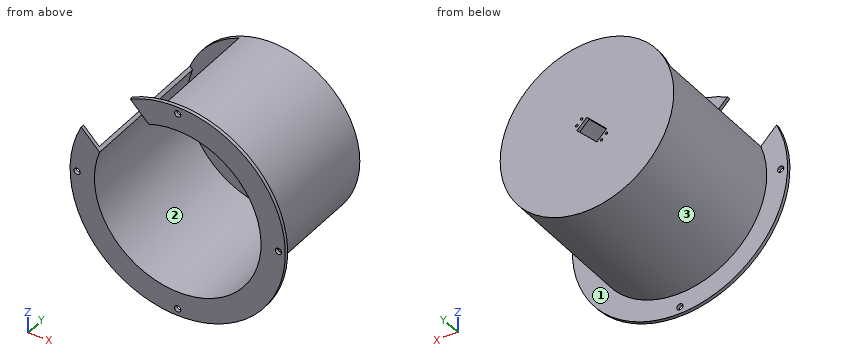
Autodesk Inventor part; units mm, degrees
ref_plane "Work Plane2" through (-109.6016, 0, 109.6016) normal (0.7071, 0, -0.7071) x (0, 1, 0)
ref_plane "XZ Plane" through (0, 0, 0) normal (0, 1, 0) x (-1, 0, 0)
ref_plane "XY Plane" through (0, 0, 0) normal (0, 0, 1) x (1, 0, 0)
sketch "Sketch1" plane through (0, 0, 0) normal (0, 1, 0) x (-1, 0, 0)
  circle A0 centre (0, 0) radius 120
  circle A1 centre (0, 0) radius 125
  circle A2 centre (0, 0) radius 155
  dimension "d0" = 240
  dimension "d1" = 250
  dimension "d2" = 310
extrude "Extrusion1" add sketch "Sketch1" along normal blind 205 contours A0 | A1 | A2
sketch "Sketch3" plane through (0, 205, 0) normal (0, 1, 0) x (1, 0, 0)
  circle A0 centre (0, 0) radius 155
  circle A1 centre (0, 0) radius 125
  dimension "d27" = 250
  dimension "d28" = 310
extrude "Extrusion3" cut sketch "Sketch3" against normal blind 200
sketch "Sketch4" plane through (0, 5, 0) normal (0, 1, 0) x (1, 0, 0)
  circle A0 centre (0, 145) radius 4.5
  circle A1 centre (0, 0) radius 155
  line L0 (0, 155) -> (0, 125)
  circle A2 centre (0, 0) radius 125
  circle A3 centre (-145, 0) radius 4.5
  line L1 (-155, 0) -> (-125, 0)
  circle A4 centre (0, -145) radius 4.5
  line L2 (0, -155) -> (0, -125)
  circle A5 centre (145, 0) radius 4.5
  line L3 (155, 0) -> (125, 0)
  dimension "d31" = 9
  dimension "d32" = 0
  dimension "d33" = 145
  dimension "d36" = 360
extrude "Extrusion4" cut sketch "Sketch4" against normal through all contours A0 L0 | L0 A0 | L3 A5 | A5 L3 | L1 A3 | A3 L1 | L2 A4 | A4 L2
sketch "Sketch5" plane through (0, 0, 0) normal (0, -1, 0) x (1, 0, 0)
  circle A0 centre (0, 0) radius 120
  dimension "d40" = 240
extrude "Extrusion5" cut sketch "Sketch5" against normal blind 200
ref_plane "Work Plane2" through (-109.6016, 0, 109.6016) normal (0.7071, 0, -0.7071) x (0, 1, 0)
ref_plane "Work Plane1" through (0, 0, 0) normal (0.7071, 0, -0.7071) x (0, 1, 0)
sketch "Sketch6" plane through (-109.6016, 0, 109.6016) normal (0.7071, 0, -0.7071) x (0, 1, 0)
  line L0 (0, -50) -> (200, -50)
  line L1 (200, -50) -> (200, 50)
  line L2 (200, 50) -> (0, 50)
  line L3 (0, 50) -> (0, -50)
  line L4 (0, 155) -> (0, -155)
  line L5 (-41, 0) -> (246, 0)
  point P0 (0, 0)
  dimension "d44" = 200
  dimension "d45" = 100
  dimension "d46" = 0
  dimension "d47" = 50
extrude "Extrusion6" cut sketch "Sketch6" along normal up to surface
sketch "Sketch7" plane through (0, 205, 0) normal (0, 1, 0) x (1, 0, 0)
  circle A0 centre (0, 0) radius 10
  line L0 (0, 0) -> (31, 0) construction
  line L1 (7.0711, 7.0711) -> (-14.2128, 28.355)
  line L2 (-14.2128, 28.355) -> (-28.355, 14.2128)
  line L3 (-28.355, 14.2128) -> (-7.0711, -7.0711)
  line L4 (-7.0711, -7.0711) -> (0.2828, -14.425)
  line L5 (-7.0711, -7.0711) -> (3.3289, -7.0711) construction
  line L6 (0.2828, -14.425) -> (14.425, -0.2828)
  line L7 (14.425, -0.2828) -> (7.0711, 7.0711)
  circle A1 centre (-28.0368, 20.9657) radius 1.75
  circle A2 centre (-20.9657, 28.0368) radius 1.75
  circle A3 centre (7.6721, -14.7432) radius 1.75
  circle A4 centre (14.7432, -7.6721) radius 1.75
  dimension "d50" = 20
  dimension "d53" = 20
  dimension "d55" = 10.4
  dimension "d56" = 45
  dimension "d57" = 30.1
  dimension "d58" = 3.5
  dimension "d61" = 5
  dimension "d65" = 10
  dimension "d68" = 50.5
  dimension "d71" = 4.55
extrude "Extrusion7" cut sketch "Sketch7" against normal through all
properties part number "mechanism_cover"
Geometry check sheet. Reference: the model listing, model coordinates, mm. Face numbers are marked on the shaded views. Give positions to 0.01 mm unless a question says otherwise; leave off trailing zeros. Loops run counter-clockwise (first coordinate to the right, second up) from the corner with the lowest first, then second, coordinate; pieces in that order, holes last. Notation, with made-up numbers: M 66,-25 L 90,-25 A12 cw 90,-18 Z; hole C 64,29 d9. An arc over 180 degrees is marked long. Answer as a JSON object with one key per item and string values. Group by question number.
Item 1: Sectioned sample at A-A on z = -145. Record the boundary of the cut face in (x, y), plus the area to 3 significant figures.
Item 2: Sectioned sample at B-B on x = 145. Record the boundary of the cut face in (y, z).
Item 3: Material ranges on L1, parallel to X at y = 2, z = 0; L2, parallel to Z at x = 0, y = 112.5, recorded low to high.
Item 4: Mould release check, pull along X, two halves, no side actions. Record for the marked faces 1, 2 and 3: pulls with the +X half, pulls with the -X half, needs draft (parallel to the pull), parting line crosses it, or undercut.
Item 5: Sectioned sample at D-D on x = -95. Record the boundary of the cut face in (y, z), plus the area to 3 significant figures.
Item 6: Sectioned sample at C-C on z = -50. Record the boundary of the cut face in (x, y), plus the area to 3 significant figures.
Item 7: Gauge pin test, flat ends, axial feed: pin 1 (2 mm diameter, centred on x = -123, z = -74, fed in from +Y); pin 2 (10 mm diameter, centred on x = 59, y = 166, fed in from -Z); pin 3 (1 mm diameter, centred on x = 54, z = 34.5, fed in from -Y). Record the tip position at first contact, or that the pin passes through.
Findings below:
{
 "1": {"outline": "M -54.77,0 L -4.5,0 L -4.5,5 L -54.77,5 Z; M 4.5,0 L 54.77,0 L 54.77,5 L 4.5,5 Z", "area": "503 mm2"},
 "2": {"outline": "M 0,-54.77 L 5,-54.77 L 5,-4.5 L 0,-4.5 Z; M 0,4.5 L 5,4.5 L 5,54.77 L 0,54.77 Z"},
 "3": {"L1": "-155 to -149.5, -140.5 to -120, 120 to 140.5, 149.5 to 155", "L2": "-125 to -120, 120 to 125"},
 "4": {"face 1": "needs draft", "face 2": "undercut", "face 3": "parting line crosses it"},
 "5": {"outline": "M 0,-122.47 L 5,-122.47 L 5,-81.24 L 205,-81.24 L 205,81.24 L 200,81.24 L 200,-73.31 L 0,-73.31 Z", "area": "2,600 mm2"},
 "6": {"outline": "M -146.71,0 L -109.09,0 L -109.09,200 L 109.09,200 L 109.09,0 L 146.71,0 L 146.71,5 L 114.56,5 L 114.56,205 L -114.56,205 L -114.56,5 L -146.71,5 Z", "area": "3,660 mm2"},
 "7": {"pin 1": "y = 5", "pin 2": "z = -112.73", "pin 3": "y = 200"}
}
